Autodesk Inventor part; units mm, degrees
ref_plane "YZ Plane" through (0, 0, 0) normal (1, 0, 0) x (0, 1, 0)
ref_plane "XZ Plane" through (0, 0, 0) normal (0, 1, 0) x (-1, 0, 0)
ref_plane "XY Plane" through (0, 0, 0) normal (0, 0, 1) x (1, 0, 0)
sketch "Szkic1" plane through (0, 0, 0) normal (0, 1, 0) x (-1, 0, 0)
  line L0 (180, 0) -> (-30, 0)
  line L1 (0, -42.9384) -> (0, 29.3231)
  line L2 (150, 10) -> (130, 10)
  line L3 (130, 10) -> (130, -10)
  line L4 (130, -10) -> (150, -10)
  line L5 (150, -10) -> (150, 10)
  line L6 (150, 10) -> (130, -10) construction
  line L7 (130, 10) -> (150, -10) construction
  circle A0 centre (140, -15) radius 1.6
  circle A1 centre (140, -15) radius 4
  line L8 (146, -10) -> (143.7732, -16.3278)
  line L9 (140, 0) -> (140, -32.6153) construction
  line L10 (134, -10) -> (136.2268, -16.3278)
  circle A2 centre (140, 15) radius 1.6
  circle A3 centre (140, 15) radius 4
  line L11 (146, 10) -> (143.7732, 16.3278)
  line L12 (134, 10) -> (136.2268, 16.3278)
  point P0 (0, 0)
  dimension "d21" = 8
  dimension "d3" = 20
  dimension "d4" = 20
  dimension "d5" = 140
  dimension "d19" = 3.2
  dimension "d20" = 15
  dimension "d22" = 12
extrude "Wyciągnięcie proste1" add sketch "Szkic1" along normal blind 35 contours L5 L4 L3 L0 | L0 L3 L2 L5
sketch "Szkic2" plane through (-130, 0, 10) normal (1, 0, 0) x (0, 0, -1)
  line L0 (10, -7) -> (10, 42)
  line L1 (24, 0) -> (-4, 0)
  line L2 (0, 35) -> (20, 35)
  line L3 (20, 35) -> (20, 25)
  line L4 (20, 25) -> (0, 25)
  line L5 (0, 25) -> (0, 35)
  line L6 (0, 35) -> (20, 25) construction
  line L7 (20, 35) -> (0, 25) construction
  line L8 (0, 0) -> (20, 0)
  point P0 (10, 0)
  point P1 (10, 30)
  point P2 (10, 0)
  dimension "d8" = 20
  dimension "d9" = 10
  dimension "d10" = 30
extrude "Wyciągnięcie proste2" add sketch "Szkic2" along normal blind 50
sketch "Szkic3" plane through (-130, 25, -10) normal (0, -1, 0) x (1, 0, 0)
  circle A0 centre (40, 10) radius 4.5
  line L0 (130, -4) -> (130, 24)
  line L1 (-50, 10) -> (160, 10)
  point P0 (130, 10)
  dimension "d13" = 9
  dimension "d14" = 90
extrude "Wyciągnięcie proste3" add sketch "Szkic3" along normal blind 10
fillet "Zaokrąglenie1" radius 1 2 edges at (-94.5, 15, 0) (-94.5, 25, 0)
fillet "Zaokrąglenie2" radius 5 13 edges at (-105, 25, 10) (-130, 12.5, 10) (-130, 12.5, -10) (-105, 25, -10) (-115, 35, 10) (-150, 17.5, -10) (-150, 17.5, 10) (-115, 35, -10) (-80, 25, 0) (-80, 35, 0) (-80, 30, -10) (-80, 30, 10) (-150, 35, 0)
extrude "Wyciągnięcie proste4" add sketch "Szkic1" along normal blind 7 contours L8 A1 L10 L4 | L2 L12 A3 L11 | A1 | A3
properties part number "uMule-uchwyt_servo"
Model file for the job. Use its own axes, mm. A direction names the side the tool comes from. Coordinates: 2 decimals unless noted, no trailing zeros. Order: outer loops, then holes, each group sorted by start corner. A loop starts at its lowest first (then second) coordinate and runs counter-clockwise, first axis right, second up. Notation, with made-up numbers: M 2,82 L 14,82 A35 ccw 14,117 Z; hole C -34,24 d5. An arc over 180 degrees is marked long. Answer as CSV lines item,"result".
(1) Pull direction X, two halves, no side cores. Call faces 5 (the cylindrical face through (-94.496, 20.056, -0.198)), 6 (the cylindrical face through (-140, 3, 19)), 7 (the flat face through (-144.9, 3.45, -13.12)), 8 (the cylindrical face through (-82, 26, -4)): +X half, -X half, draft (parallel to the pull), parting line (faces both ways), or undercut.
Geometry says:
face 5,"undercut"
face 6,"parting line"
face 7,"-X half"
face 8,"+X half"
(2) Wall check: line 1 along Z through (x, y) = (-140, 3); line 2 along X through (y, z) = (16, 0); line 3 along Y through (x, z) = (-101, 0.5). Give the ranges that are in metal, low to high.
Geometry says:
line 1,"z = -19 to -16.6, -13.4 to 13.4, 16.6 to 19"
line 2,"x = -150 to -130, -94.5 to -85.5"
line 3,"y = 25 to 35"
(3) Band-saw the part on B-B, the plane z = -15. List the corners of the cut face in (x, y).
Geometry says:
outline,"M -144.24,0 L -141.6,0 L -141.6,7 L -144.24,7 Z; M -138.4,0 L -135.76,0 L -135.76,7 L -138.4,7 Z"
(4) Band-saw the part on A-A, the plane x = -140. List the corners of the cut face in (y, z).
Geometry says:
outline,"M 0,-19 L 7,-19 L 7,-16.6 L 0,-16.6 Z; M 0,-13.4 L 7,-13.4 L 7,-10 L 30,-10 A5 ccw 35,-5 L 35,5 A5 ccw 30,10 L 7,10 L 7,13.4 L 0,13.4 Z; M 0,16.6 L 7,16.6 L 7,19 L 0,19 Z"
(5) Band-saw the part on C-C, the plane y = 8. List the corners of the cut face in (x, z), then the cut area to 3 significant figures.
Geometry says:
outline,"M -150,-5 A5 ccw -145,-10 L -135,-10 A5 ccw -130,-5 L -130,5 A5 ccw -135,10 L -145,10 A5 ccw -150,5 Z"
area,"379 mm2"
(6) 3-axis set-ups, long thin cutter, end or side, ignore diameter. For faces 1 (the flat face through (-140, 18, 10)), 2 (the cylindrical face through (-86, 26, -8)), 3 (the cylindrical face through (-86, 27, 9)), 4 (the flat face through (-90, 15, 0)): which of +Z, -Z, +X, -X, +Y, -Y reach the whole face in a straight line?
Geometry says:
face 1,"+Z, +X, -X, +Y"
face 2,"-Z, +X, -Y"
face 3,"+Z, +X, -Y"
face 4,"+Z, -Z, +X, -Y"
(7) Flat gauge pins, fed straight in: pin 1 (18.5 mm diameter, centred on x = -101.5, y = 20.5, fed in from +Z); pin 2 (3.5 mm diameter, centred on x = -140, z = -15, fed in from +Y); pin 3 (12 mm diameter, centred on x = -132.5, y = 27, fed in from -Z); pin 4 (1.5 mm diameter, centred on x = -142, z = 8.5, fed in from -Y). Where does each tip first touch, or does it go through?
Geometry says:
pin 1,"stops at z = 9.99"
pin 2,"stops at y = 7"
pin 3,"stops at z = -10"
pin 4,"stops at y = 0"
